Can you work these out from the drawing? Everything is in mm from the part's minimum corner. Coordinates: 2 decimals unless noted, no trailing zeros. Order: outer loops, then holes, each group sorted by start corner. A loop starts at its lowest first (then second) coordinate and runs counter-clockwise, first axis right, second up. Notation, with made-up numbers: (25, -40) -> (66, -40) arc R32 cw to (66, -9) -> close; hole circle Ø9 at (78, -15.5). An arc over 180 degrees is marked (long way). Put each result on its own line as item: value. Start each with the question number.
Q1. Will these pins go through, and if not, where does the flat tip stop? pin 1 (2.5 mm diameter, centred on x = 1.5, y = 103, fed in from +Z); pin 2 (10 mm diameter, centred on y = 59, z = 313, fed in from -X); pin 3 (6 mm diameter, centred on x = 9, y = 91.5, fed in from +Z); pin 4 (4 mm diameter, centred on y = 77.5, z = 189, fed in from +X).
Q2. If we section it at C-C (z = 210): Please give me the cut outline in (x, y), and give its area (3 significant figures).
Q3. If we section it at D-D (y = 120.5): Please give me the cut outline in (x, z), and give its area (3 significant figures).
Q4. If we section it at A-A (x = 7): Please give me the cut outline in (y, z).
Q5. If we section it at B-B (y = 65.5): Please give me the cut outline in (x, z).
Q6. Please list where these lines run through material, in increasing order: line 1 along Z through (x, y) = (4.75, 90); line 2 along X through (y, z) = (87, 70.5); line 3 along Z through (x, y) = (7.25, 191.5).
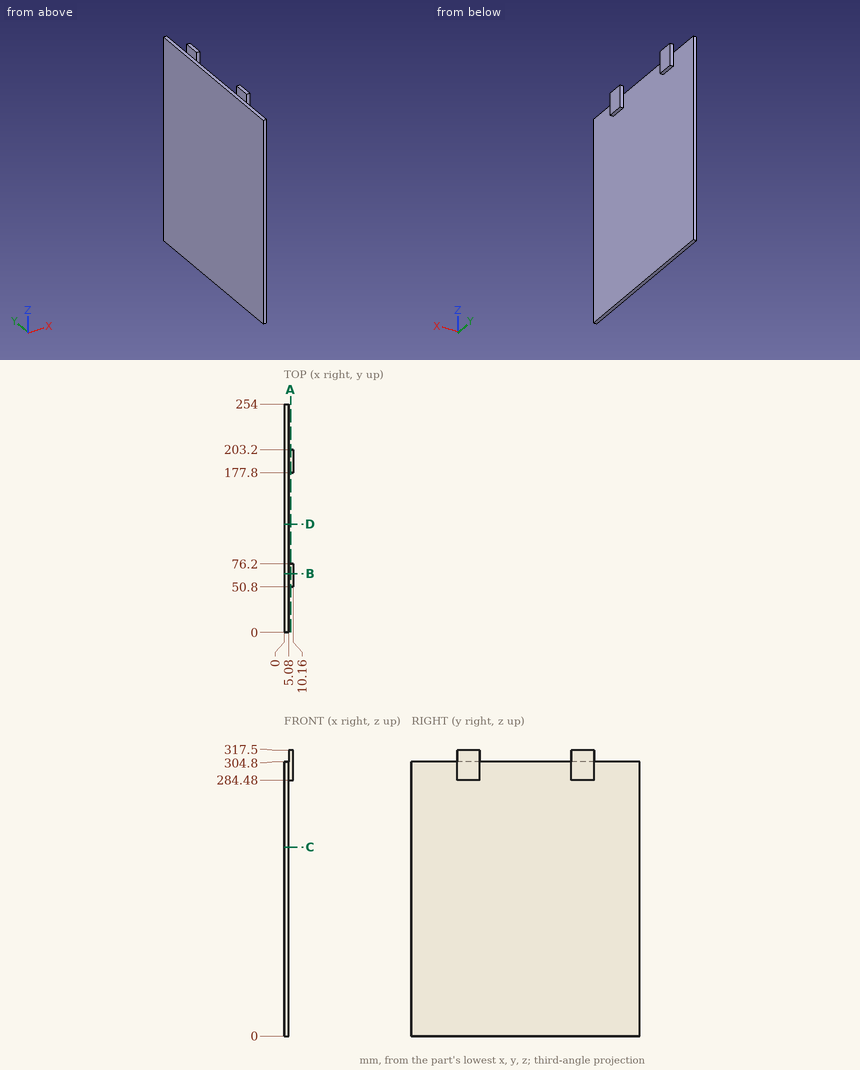
The answers:
1. pin 1: z = 304.8
1. pin 2: x = 5.08
1. pin 3: through
1. pin 4: x = 5.08
2. outline: (0, 0) -> (5.08, 0) -> (5.08, 254) -> (0, 254) -> close
2. area: 1,290 mm^2
3. outline: (0, 0) -> (5.08, 0) -> (5.08, 304.8) -> (0, 304.8) -> close
3. area: 1,550 mm^2
4. outline: (50.8, 284.48) -> (76.2, 284.48) -> (76.2, 317.5) -> (50.8, 317.5) -> close; (177.8, 284.48) -> (203.2, 284.48) -> (203.2, 317.5) -> (177.8, 317.5) -> close
5. outline: (0, 0) -> (5.08, 0) -> (5.08, 284.48) -> (10.16, 284.48) -> (10.16, 317.5) -> (5.08, 317.5) -> (5.08, 304.8) -> (0, 304.8) -> close
6. line 1: 0 to 304.8
6. line 2: 0 to 5.08
6. line 3: 284.48 to 317.5
